from build123d import *

# Parameters (mm, degrees)
BOSS_EXTRUDE1_DEPTH = 20
SKETCH2_R           = 2
CUT_EXTRUDE1_DEPTH  = 2.5
SKETCH3_R           = 6.5
BOSS_EXTRUDE2_DEPTH = 2


with BuildPart() as part:
    # Sketch1 → Boss-Extrude1 (new body)
    with BuildSketch(Plane(origin=(0, 0, 0), x_dir=(1, 0, 0), z_dir=(0, 1, 0))):
        Polygon((11.5, 20), (19, 20), (19, -20), (11.5, -20), (11.5, -27), (9, -27), (9, -20), (-19, -20), (-19, 20), (9, 20), (9, 27), (11.5, 27), align=None)
    extrude(amount=BOSS_EXTRUDE1_DEPTH)

    # Sketch2 → Cut-Extrude1 (cut)
    with BuildSketch(Plane(origin=(11.5, 0, 0), x_dir=(0, 0, -1), z_dir=(1, 0, 0))):
        with Locations((-24.5, 15)):
            Circle(SKETCH2_R)
        with Locations((-24.5, 5)):
            Circle(SKETCH2_R)
        with Locations((24.5, 5)):
            Circle(SKETCH2_R)
        with Locations((24.5, 15)):
            Circle(SKETCH2_R)
    extrude(amount=-CUT_EXTRUDE1_DEPTH, mode=Mode.SUBTRACT)

    # Sketch3 → Boss-Extrude2 (add)
    with BuildSketch(Plane(origin=(19, 0, 0), x_dir=(0, 0, -1), z_dir=(1, 0, 0))):
        with Locations(Location((10, 10, 0), (0, 0, 180))):
            Circle(SKETCH3_R)
    extrude(amount=BOSS_EXTRUDE2_DEPTH)


solid = part.part
The model under review builds one solid part; all positions refer to its coordinate system, in mm. A direction names the side the tool comes from. Give positions to 0.01 mm unless a question says otherwise; leave off trailing zeros. Loops run counter-clockwise (first coordinate to the right, second up) from the corner with the lowest first, then second, coordinate; pieces in that order, holes last. Notation, with made-up numbers: (39, 81) -> (86, 81) arc R14 cw to (86, 92) -> close; hole circle Ø4 at (-13.5, -27). An arc over 180 degrees is marked (long way). Write each question's results on one line, items separated by ' | '.
1) Insertion check: pin 1 Ø4 at (x, y) = (16.5, 11) entering from -Z; pin 2 Ø3.5 at (y, z) = (12, 23) entering from +X; pin 3 Ø4 at (x, y) = (-14, 3) entering from +Z. Each pin has a flat end and moves straight along its axis. Give the tip position at first contact, or say it passes through.
Conclusion:
pin 1: stops at z = -20 | pin 2: stops at x = 11.5 | pin 3: stops at z = 20
2) Take a section at D-D, the plane y = 15. Give the boundary of the cut face in (x, z).
Conclusion:
outline: (-19, -20) -> (9, -20) -> (9, -22.5) -> (11.5, -22.5) -> (11.5, -20) -> (19, -20) -> (19, -14.15) -> (21, -14.15) -> (21, -5.85) -> (19, -5.85) -> (19, 20) -> (11.5, 20) -> (11.5, 22.5) -> (9, 22.5) -> (9, 20) -> (-19, 20) -> close; (9, -27) -> (11.5, -27) -> (11.5, -26.5) -> (9, -26.5) -> close; (9, 26.5) -> (11.5, 26.5) -> (11.5, 27) -> (9, 27) -> close
3) Draft analysis for pull direction Y (two halves, no side actions). For faces 1 (the face through (10.268, 16.352, 25.974)), 2 (the face through (10.268, 5.088, -22.502)), 3 (the face through (0, 20, 0)), 4 (the face through (11.5, 10, 23)), state which applies: pulls with the +Y half, pulls with the -Y half, needs draft (parallel to the pull), parting line crosses it, or undercut.
Conclusion:
face 1: undercut | face 2: undercut | face 3: pulls with the +Y half | face 4: needs draft
4) Take a section at A-A, the plane z = 24.5. Give the boundary of the cut face in (x, y), plus the area to 3 significant figures.
Conclusion:
outline: (9, 0) -> (11.5, 0) -> (11.5, 3) -> (9, 3) -> close; (9, 7) -> (11.5, 7) -> (11.5, 13) -> (9, 13) -> close; (9, 17) -> (11.5, 17) -> (11.5, 20) -> (9, 20) -> close | area: 30.0 mm^2
5) Take a section at C-C, the plane z = -10. Give the boundary of the cut face in (x, y).
Conclusion:
outline: (-19, 0) -> (19, 0) -> (19, 3.5) -> (21, 3.5) -> (21, 16.5) -> (19, 16.5) -> (19, 20) -> (-19, 20) -> close
6) Take a section at B-B, the plane y = 10. Give the boundary of the cut face in (x, z), plus the area to 3 significant figures.
Conclusion:
outline: (-19, -20) -> (9, -20) -> (9, -27) -> (11.5, -27) -> (11.5, -20) -> (19, -20) -> (19, -16.5) -> (21, -16.5) -> (21, -3.5) -> (19, -3.5) -> (19, 20) -> (11.5, 20) -> (11.5, 27) -> (9, 27) -> (9, 20) -> (-19, 20) -> close | area: 1,580 mm^2
7) Tool access review of faces 5 (the face through (9, 10, -23)), 6 (the face through (9, 10, 24)), 7 (the face through (11.5, 10, -24)), 8 (the face through (15, 10, 20)): name each direction out of +Z, -Z, +X, -X, +Y, -Y from which nothing blocks a thin tool from reaching the whole face with its end or side.
Conclusion:
face 5: -Z, -X, +Y, -Y | face 6: +Z, -X, +Y, -Y | face 7: -Z, +X, +Y, -Y | face 8: +Z, +X, +Y, -Y
8) For line 1 along Y through (x, z) = (10.55, -24.5); line 2 along Z through (x, y) = (-9, 15.5); line 3 along X through (y, z) = (16, 12), list the stretches that pass through material, from the lowest coordinate up. Write a range as from..to.
Conclusion:
line 1: y = 0..3, 7..13, 17..20 | line 2: z = -20..20 | line 3: x = -19..19
